The drawing under review shows one solid part. Ordinate dimensions are in mm from its lowest x, y, z. A direction names the side the tool comes from. Round coordinates to 2 decimals unless told otherwise and drop trailing zeros. Write each loop counter-clockwise with the first axis right and the second up, starting at its lowest first coordinate (ties: lowest second). Pieces come first, ordered by that corner, then holes.
Item 1: Draft analysis for pull direction Z (two halves, no side actions). For the marked faces 1, 2 and 3, state which applies: +Z half, -Z half, draft (parallel to the pull), parting line (faces both ways), or undercut.
Item 2: To check wall thickness, follow L1, parallel to Y at x = 9, z = 4; L2, parallel to X at y = 1.2, z = 5.5; L3, parallel to Z at x = 4, y = 2.5. State the ranges of each line that lie inside material, in increasing order.
Item 3: Add section C-C (x = 4). Give the boundary of the cut face in (y, z).
Item 4: Add section D-D (z = 16.75). Give the boundary of the cut face in (x, y).
Item 5: Machinability: for the marked faces 4, 5 and 6, which of the approach directions +Z, -Z, +X, -X, +Y, -Y give a long, thin tool a straight path to every point of the face, cutting with its end or side? Answer none if there is none.
Item 6: Add section A-A (y = 1.85). Give the boundary of the cut face in (x, z), plus the area to 4 significant figures.
Item 7: Clearance check with flat-ended pins moving along their axes: pin 1 Ø2 at (y, z) = (1, 3) entering from -X; pin 2 Ø1.5 at (x, y) = (43.5, 2.5) entering from +Z; pin 3 Ø0.8 at (y, z) = (3, 6.5) entering from +X; pin 4 Ø2.5 at (x, y) = (43.5, 4) entering from -Z. State where each tip first meets the part, or that it passes through.
Item 8: Add section B-B (z = 10.5). Give the boundary of the cut face in (x, y).
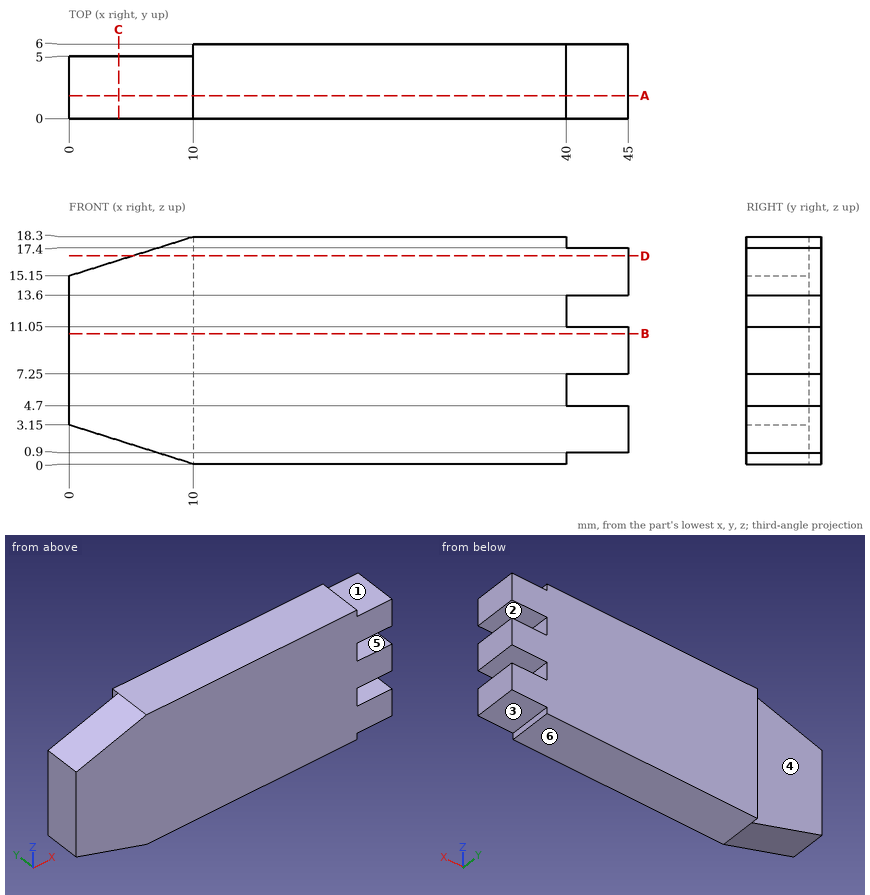
Numbers:
1. face 1: +Z half
1. face 2: undercut
1. face 3: -Z half
2. L1: y = 0 to 5
2. L2: x = 0 to 40
2. L3: z = 1.89 to 16.41
3. outline: (0, 1.89) - (5, 1.89) - (5, 16.41) - (0, 16.41) - close
4. outline: (5.08, 0) - (45, 0) - (45, 6) - (10, 6) - (10, 5) - (5.08, 5) - close
5. face 4: +Z, -Z, -X, +Y
5. face 5: +X, +Y, -Y
5. face 6: -Z, +X, -X, +Y, -Y
6. outline: (0, 3.15) - (10, 0) - (40, 0) - (40, 0.9) - (45, 0.9) - (45, 4.7) - (40, 4.7) - (40, 7.25) - (45, 7.25) - (45, 11.05) - (40, 11.05) - (40, 13.6) - (45, 13.6) - (45, 17.4) - (40, 17.4) - (40, 18.3) - (10, 18.3) - (0, 15.15) - close
6. area: 757.5 mm2
7. pin 1: stops at x = 0
7. pin 2: stops at z = 17.4
7. pin 3: stops at x = 40
7. pin 4: stops at z = 0.9
8. outline: (0, 0) - (45, 0) - (45, 6) - (10, 6) - (10, 5) - (0, 5) - close
